```python
from build123d import *

# Parameters (mm, degrees)
SKETCH_2_R                 = 1.85
EXTRUDE_1_DEPTH            = 5.6
SKETCH_3_R                 = 2.95
CUT_EXTRUDE_1_DEPTH        = 3.6
SKETCH_4_W                 = 8
SKETCH_4_H                 = 23.2
EXTRUDE_2_DEPTH            = 7.2
SKETCH_5_R                 = 2.4
CUT_EXTRUDE_2_DEPTH        = 29.8
CUT_EXTRUDE_2_DEPTH_BACK   = 29.8
FILLET_1_R                 = 3.6
SKETCH_6_R                 = 3.1
CUT_EXTRUDE_3_DEPTH        = 0.8
MIRROR_2_COPY_1_SKETCH_R   = 3.1
MIRROR_2_COPY_1_DEPTH      = 0.8
CUT_EXTRUDE_4_DEPTH        = 6.6
SKETCH_8_W                 = 19
SKETCH_8_H                 = 18
CUT_EXTRUDE_5_DEPTH        = 4
FILLET_3_R                 = 2
FILLET_4_R                 = 0.1
FILLET_5_R                 = 1
CHAMFER_1_SIZE             = 1
FILLET_5_OF_MIRROR_3_R     = 1
CHAMFER_1_OF_MIRROR_3_SIZE = 1
CHAMFER_2_SIZE             = 1.2
SKETCH_9_W                 = 0.1
SKETCH_9_H                 = 1.6
EXTRUDE_3_DEPTH            = 8


with BuildPart() as part:
    # ｽｹｯﾁ2 → ﾎﾞｽ - 押し出し1 (new body)
    with BuildSketch(Plane.XY):
        with BuildLine():
            Line((-12, 11.6), (-26.202629265, 4.264788895))
            ThreePointArc((-26.202629265, 4.264788895), (-28.8, 0), (-26.202629265, -4.264788895))
            Line((-26.202629265, -4.264788895), (-12, -11.6))
            Line((-12, -11.6), (12, -11.6))
            Line((12, -11.6), (26.202629265, -4.264788895))
            ThreePointArc((26.202629265, -4.264788895), (28.8, 0), (26.202629265, 4.264788895))
            Line((26.202629265, 4.264788895), (12, 11.6))
            Line((12, 11.6), (-12, 11.6))
        make_face()
        with Locations((-24, 0)):
            Circle(SKETCH_2_R, mode=Mode.SUBTRACT)
        with Locations((24, 0)):
            Circle(SKETCH_2_R, mode=Mode.SUBTRACT)
    extrude(amount=EXTRUDE_1_DEPTH)

    # ｽｹｯﾁ3 → ｶｯﾄ - 押し出し1 (cut)
    with BuildSketch(Plane(origin=(0, 0, 0), x_dir=(-1, 0, 0), z_dir=(0, 0, -1))):
        with Locations((-24, 0)):
            Circle(SKETCH_3_R)
        with Locations((24, 0)):
            Circle(SKETCH_3_R)
    extrude(amount=-CUT_EXTRUDE_1_DEPTH, mode=Mode.SUBTRACT)

    # ｽｹｯﾁ4 → ﾎﾞｽ - 押し出し2 (add)
    with BuildSketch(Plane(origin=(0, 0, 0), x_dir=(-1, 0, 0), z_dir=(0, 0, -1))):
        with Locations((-8, 0)):
            Rectangle(SKETCH_4_W, SKETCH_4_H)
        with Locations((8, 0)):
            Rectangle(SKETCH_4_W, SKETCH_4_H)
    extrude(amount=EXTRUDE_2_DEPTH)

    # ｽｹｯﾁ5 → ｶｯﾄ - 押し出し2 (cut, two sides)
    with BuildSketch(Plane(origin=(0, 0, 0), x_dir=(0, 0, -1), z_dir=(1, 0, 0))) as cut_extrude_2_sk:
        with Locations((3.6, 8)):
            Circle(SKETCH_5_R)
        with Locations((3.6, -8)):
            Circle(SKETCH_5_R)
        with BuildLine():
            Line((2.8, 2.2627417), (2.8, 0.8))
            Line((2.8, 0.8), (1.3372583, 0.8))
            ThreePointArc((1.3372583, 0.8), (1.2, 0), (1.3372583, -0.8))
            Line((1.3372583, -0.8), (2.8, -0.8))
            Line((2.8, -0.8), (2.8, -2.2627417))
            ThreePointArc((2.8, -2.2627417), (3.6, -2.4), (4.4, -2.2627417))
            Line((4.4, -2.2627417), (4.4, -0.8))
            Line((4.4, -0.8), (5.8627417, -0.8))
            ThreePointArc((5.8627417, -0.8), (6, 0), (5.8627417, 0.8))
            Line((5.8627417, 0.8), (4.4, 0.8))
            Line((4.4, 0.8), (4.4, 2.2627417))
            ThreePointArc((4.4, 2.2627417), (3.6, 2.4), (2.8, 2.2627417))
        make_face()
    extrude(amount=CUT_EXTRUDE_2_DEPTH, mode=Mode.SUBTRACT)
    extrude(cut_extrude_2_sk.sketch, amount=-CUT_EXTRUDE_2_DEPTH_BACK, mode=Mode.SUBTRACT)

    # ﾌｨﾚｯﾄ1
    fillet_1_edges = [part.edges().sort_by_distance(p)[0] for p in [
        (8, -11.6, -7.2),
        (8, 11.6, -7.2),
        (-8, -11.6, -7.2),
        (-8, 11.6, -7.2),
    ]]
    fillet(fillet_1_edges, radius=FILLET_1_R)

    # ｽｹｯﾁ6 → ｶｯﾄ - 押し出し3 (cut)
    with BuildSketch(Plane.ZY.offset(-4)):
        with Locations((-3.6, 8)):
            Circle(SKETCH_6_R)
        with Locations((-3.6, -8)):
            Circle(SKETCH_6_R)
    cut_extrude_3 = extrude(amount=-CUT_EXTRUDE_3_DEPTH, mode=Mode.SUBTRACT)

    # ﾐﾗｰ1: ｶｯﾄ - 押し出し3 across plane
    add(cut_extrude_3.mirror(Plane(origin=(8, 0, 0), x_dir=(0, 0, 1), z_dir=(1, 0, 0))), mode=Mode.SUBTRACT)

    # ﾐﾗｰ2: ｶｯﾄ - 押し出し3 across plane
    add(cut_extrude_3.mirror(Plane(origin=(0, 0, 0), x_dir=(0, 0, 1), z_dir=(1, 0, 0))), mode=Mode.SUBTRACT)

    # ﾐﾗｰ2 copy 1 sketch → ﾐﾗｰ2 copy 1 (cut)
    with BuildSketch(Plane.ZY.offset(12)):
        with Locations((-3.6, 8)):
            Circle(MIRROR_2_COPY_1_SKETCH_R)
        with Locations((-3.6, -8)):
            Circle(MIRROR_2_COPY_1_SKETCH_R)
    extrude(amount=-MIRROR_2_COPY_1_DEPTH, mode=Mode.SUBTRACT)

    # ｽｹｯﾁ7 → ｶｯﾄ - 押し出し4 (cut, through all)
    with BuildSketch(Plane(origin=(0, 0, 0), x_dir=(-1, 0, 0), z_dir=(0, 0, -1))):
        Polygon((-19, 4.608234267), (-19, -4.608234267), (-15, -6.6741084), (-15, 6.6741084), align=None)
    cut_extrude_4 = extrude(amount=-CUT_EXTRUDE_4_DEPTH, mode=Mode.SUBTRACT)

    # ｽｹｯﾁ8 → ｶｯﾄ - 押し出し5 (cut)
    with BuildSketch(Plane.XY.offset(5.6)):
        Rectangle(SKETCH_8_W, SKETCH_8_H)
    extrude(amount=-CUT_EXTRUDE_5_DEPTH, mode=Mode.SUBTRACT)

    # ﾌｨﾚｯﾄ3
    fillet_3_edges = [part.edges().sort_by_distance(p)[0] for p in [
        (-9.5, -9, 3.6),
        (-9.5, 9, 3.6),
        (9.5, 9, 3.6),
        (9.5, -9, 3.6),
    ]]
    fillet(fillet_3_edges, radius=FILLET_3_R)

    # ﾌｨﾚｯﾄ4
    fillet_4_edges = [part.edges().sort_by_distance(p)[0] for p in [
        (4, 0, -7.2),
        (4, 11.6, -1.8),
        (4, -11.6, -1.8),
        (4, 10.545584412, -6.145584412),
        (4, -10.545584412, -6.145584412),
        (-4, -11.6, -1.8),
        (-4, 0, -7.2),
        (-4, 11.6, -1.8),
        (-4, 10.545584412, -6.145584412),
        (-4, -10.545584412, -6.145584412),
    ]]
    fillet(fillet_4_edges, radius=FILLET_4_R)

    # ﾌｨﾚｯﾄ5
    fillet_5_edges = [part.edges().sort_by_distance(p)[0] for p in [
        (19, 4.608234267, 2.8),
        (19, -4.608234267, 2.8),
    ]]
    fillet(fillet_5_edges, radius=FILLET_5_R)

    # 面取り1
    chamfer_1_edges = [part.edges().sort_by_distance(p)[0] for p in [
        (16.729440548, 5.780906776, 0),
        (15, 0, 0),
        (16.729440548, -5.780906776, 0),
        (19, 0, 0),
        (18.854072918, -4.519360763, 0),
        (18.854072918, 4.519360763, 0),
    ]]
    chamfer(chamfer_1_edges, length=CHAMFER_1_SIZE)

    # ﾐﾗｰ3: ｶｯﾄ - 押し出し4 across plane
    add(cut_extrude_4.mirror(Plane(origin=(0, 0, 0), x_dir=(0, 0, 1), z_dir=(1, 0, 0))), mode=Mode.SUBTRACT)

    # ﾌｨﾚｯﾄ5 of ﾐﾗｰ3
    fillet_5_of_mirror_3_edges = [part.edges().sort_by_distance(p)[0] for p in [
        (-19, 4.608234267, 2.8),
        (-19, -4.608234267, 2.8),
    ]]
    fillet(fillet_5_of_mirror_3_edges, radius=FILLET_5_OF_MIRROR_3_R)

    # 面取り1 of ﾐﾗｰ3
    chamfer_1_of_mirror_3_edges = [part.edges().sort_by_distance(p)[0] for p in [
        (-16.729440548, 5.780906776, 0),
        (-15, 0, 0),
        (-16.729440548, -5.780906776, 0),
        (-19, 0, 0),
        (-18.854072918, -4.519360763, 0),
        (-18.854072918, 4.519360763, 0),
    ]]
    chamfer(chamfer_1_of_mirror_3_edges, length=CHAMFER_1_OF_MIRROR_3_SIZE)

    # 面取り2
    chamfer_2_edges = [part.edges().sort_by_distance(p)[0] for p in [
        (-19.101314633, -7.932394448, 0),
        (-28.8, 0, 0),
        (-19.101314633, 7.932394448, 0),
        (19.101314633, 7.932394448, 0),
        (28.8, 0, 0),
        (19.101314633, -7.932394448, 0),
    ]]
    chamfer(chamfer_2_edges, length=CHAMFER_2_SIZE)

    # ｽｹｯﾁ9 → ﾎﾞｽ - 押し出し3 (add)
    with BuildSketch(Plane(origin=(12, 0, 0), x_dir=(0, 0, -1), z_dir=(1, 0, 0))):
        with Locations((4.45, 0)):
            Rectangle(SKETCH_9_W, SKETCH_9_H)
    extrude_3 = extrude(amount=-EXTRUDE_3_DEPTH)

    # ﾐﾗｰ4: ﾎﾞｽ - 押し出し3 across plane
    add(extrude_3.mirror(Plane(origin=(0, 0, 0), x_dir=(0, 0, 1), z_dir=(1, 0, 0))))


solid = part.part
```
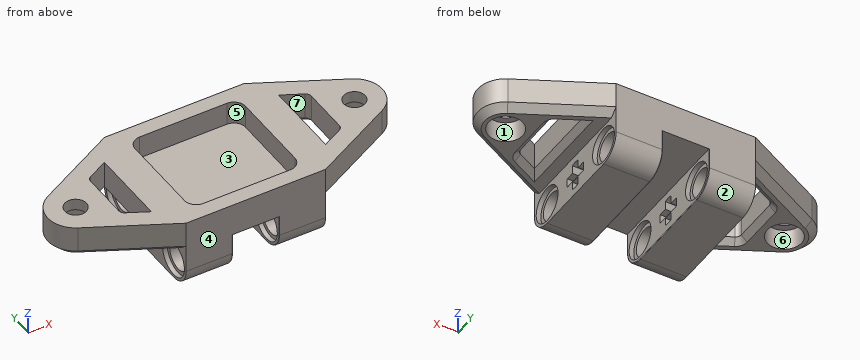
Design review of the part built by this model. Coordinates are the model's own, in mm. Face numbers are marked on the shaded views. A direction names the side the tool comes from. Coordinates: 2 decimals unless noted, no trailing zeros. Order: outer loops, then holes, each group sorted by start corner. A loop starts at its lowest first (then second) coordinate and runs counter-clockwise, first axis right, second up. Notation, with made-up numbers: (-2, 89) - (32, 89) arc R15 cw to (32, 107) - close; hole circle Ø8 at (66, -13). An arc over 180 degrees is marked (long way). Answer in a Markdown table with one row per item.
(1) Consider section B-B on z = 4.75. Give the number of separate pieces and of enclosed holes in the cut face, plus the area to 3 significant figures.
Checked values:
| item | result |
|---|---|
| separate pieces | 1 |
| enclosed holes | 5 |
| area | 589 mm^2 |
(2) Wall thickness on line 1 along Y through (x, z) = (-4.35, -3.6); line 2 along X through (y, z) = (-1.75, -6.5); line 3 along Y through (x, z) = (1.5, 2.5): over which ranges is each line inside the solid? List them lowest first. Write a range as from..to.
Checked values:
| item | result |
|---|---|
| line 1 | -11.6..-11.1, -4.9..-2.4, 2.4..4.9, 11.1..11.6 |
| line 2 | -12..-4, 4..12 |
| line 3 | -11.6..-9, 9..11.6 |
(3) Consider section A-A on x = -23. State the section outline as (y, z) points.
Checked values:
| item | result |
|---|---|
| outline | (-5.92, 1.2) - (-4.57, 0) - (-2.78, 0) - (-2.78, 3.6) - (-1.56, 3.6) - (-1.56, 5.6) - (-5.92, 5.6) - close; (1.56, 3.6) - (2.78, 3.6) - (2.78, 0) - (4.57, 0) - (5.92, 1.2) - (5.92, 5.6) - (1.56, 5.6) - close |
(4) For the marked faces 5, 6 and 7, list the 3-axis set-ups (+Z, -Z, +X, -X, +Y, -Y) from which the entire face can be reached by the end or side of a thin tool; tool diameter is ignored.
Checked values:
| item | result |
|---|---|
| face 5 | +Z |
| face 6 | -Z |
| face 7 | +Z, -Z |
(5) The part is to be moulded in two halves that separate along Y. For the marked faces 1, 2, 3 and 4, say which applies: released by +Y, released by -Y, zero draft, split by the parting line, or undercut.
Checked values:
| item | result |
|---|---|
| face 1 | undercut |
| face 2 | released by +Y |
| face 3 | undercut |
| face 4 | released by -Y |
(6) Consider section C-C on x = -3. State the section outline as (y, z) points, plus the area to 3 significant figures.
Checked values:
| item | result |
|---|---|
| outline | (-11.6, 0) - (11.6, 0) - (11.6, 5.6) - (9, 5.6) - (9, 1.6) - (-9, 1.6) - (-9, 5.6) - (-11.6, 5.6) - close |
| area | 57.9 mm^2 |
(7) Clearance check with flat-ended pins moving along their axes: pin 1 (7 mm diameter, centred on y = 8, z = -3.6, fed in from +X); pin 2 (4.5 mm diameter, centred on x = -23, y = 2, fed in from -Z); pin 3 (12 mm diameter, centred on x = -17.5, y = -7.5, fed in from -Z); pin 4 (1.5 mm diameter, centred on x = 4, y = 6.5, fed in from +Z). State where each tip first meets the part, or that it passes through.
Checked values:
| item | result |
|---|---|
| pin 1 | x = 12 |
| pin 2 | z = 0 |
| pin 3 | z = -7.2 |
| pin 4 | z = 1.6 |
